The listing builds one solid part. Answer for the finished solid, in the listing's coordinates (mm). Face numbers are marked on the shaded views. Give positions to 0.01 mm unless a question says otherwise; leave off trailing zeros. Loops run counter-clockwise (first coordinate to the right, second up) from the corner with the lowest first, then second, coordinate; pieces in that order, holes last.
Item 1: Consider line 1 along X through (y, z) = (-5.25, -43); line 2 along Z through (x, y) = (9, 8.5); line 3 along Y through (x, z) = (12.5, 45.5). Determine where each line is inside the solid, lowest interval first.
Item 2: The mould has two halves that part along X. Classify the marked faces 1, 2 and 3: pulls with the +X half, pulls with the -X half, needs draft (parallel to the pull), parting line crosses it, or undercut.
Item 3: Section A-A, the plane z = -24 is taken. Give the vertices of the cut face in (x, y).
Item 4: Section B-B, the plane x = -13 is taken. Give the vertices of the cut face in (y, z), and give its area (3 significant figures).
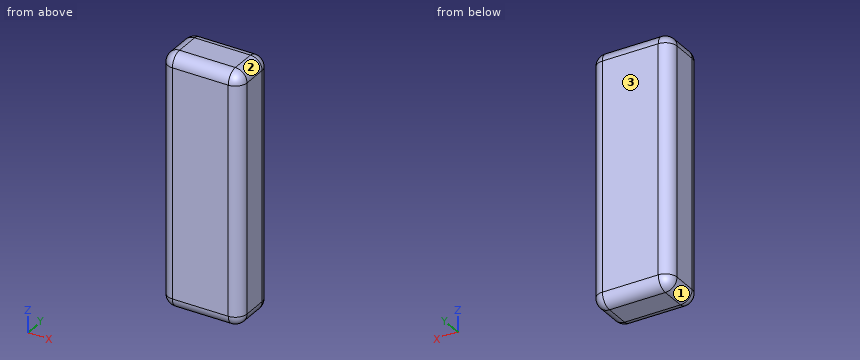
from build123d import *

# Parameters (mm, degrees)
ESQUISSE1_W             = 34
ESQUISSE1_H             = 108
BOSS_EXTRU_1_DEPTH      = 10.5
BOSS_EXTRU_1_DEPTH_BACK = 10.05
CONG_1_R                = 5
CONG_2_R                = 5


with BuildPart() as part:
    # Esquisse1 → Boss.-Extru.1 (new body, two sides)
    with BuildSketch(Plane(origin=(0, 0, 0), x_dir=(1, 0, 0), z_dir=(0, 1, 0))) as boss_extru_1_sk:
        Rectangle(ESQUISSE1_W, ESQUISSE1_H)
    extrude(amount=BOSS_EXTRU_1_DEPTH)
    extrude(boss_extru_1_sk.sketch, amount=-BOSS_EXTRU_1_DEPTH_BACK)

    # Congé1
    cong_1_edges = [part.edges().sort_by_distance(p)[0] for p in [
        (17, 0.225, 54),
        (-17, 0.225, 54),
        (-17, 0.225, -54),
        (17, 0.225, -54),
    ]]
    fillet(cong_1_edges, radius=CONG_1_R)

    # Congé2
    cong_2_edges = [part.edges().sort_by_distance(p)[0] for p in [
        (17, 10.5, 0),
        (17, -10.05, 0),
        (0, 10.5, -54),
        (-17, 10.5, 0),
        (0, 10.5, 54),
        (15.535533906, 10.5, 52.535533906),
        (-15.535533906, 10.5, 52.535533906),
        (-15.535533906, 10.5, -52.535533906),
        (15.535533906, 10.5, -52.535533906),
        (0, -10.05, -54),
        (0, -10.05, 54),
        (-17, -10.05, 0),
        (15.535533906, -10.05, 52.535533906),
        (-15.535533906, -10.05, 52.535533906),
        (-15.535533906, -10.05, -52.535533906),
        (15.535533906, -10.05, -52.535533906),
    ]]
    fillet(cong_2_edges, radius=CONG_2_R)


solid = part.part
Worked answers:
1. line 1: x = -17 to 17
1. line 2: z = -53 to 53
1. line 3: y = -10.02 to 10.47
2. face 1: pulls with the -X half
2. face 2: pulls with the +X half
2. face 3: needs draft
3. outline: (-17, -5.05) arc R5 ccw to (-12, -10.05) - (12, -10.05) arc R5 ccw to (17, -5.05) - (17, 5.5) arc R5 ccw to (12, 10.5) - (-12, 10.5) arc R5 ccw to (-17, 5.5) - close
4. outline: (-9.95, -49) arc R4.9 ccw to (-5.05, -53.9) - (5.5, -53.9) arc R4.9 ccw to (10.4, -49) - (10.4, 49) arc R4.9 ccw to (5.5, 53.9) - (-5.05, 53.9) arc R4.9 ccw to (-9.95, 49) - close
4. area: 2,170 mm2
